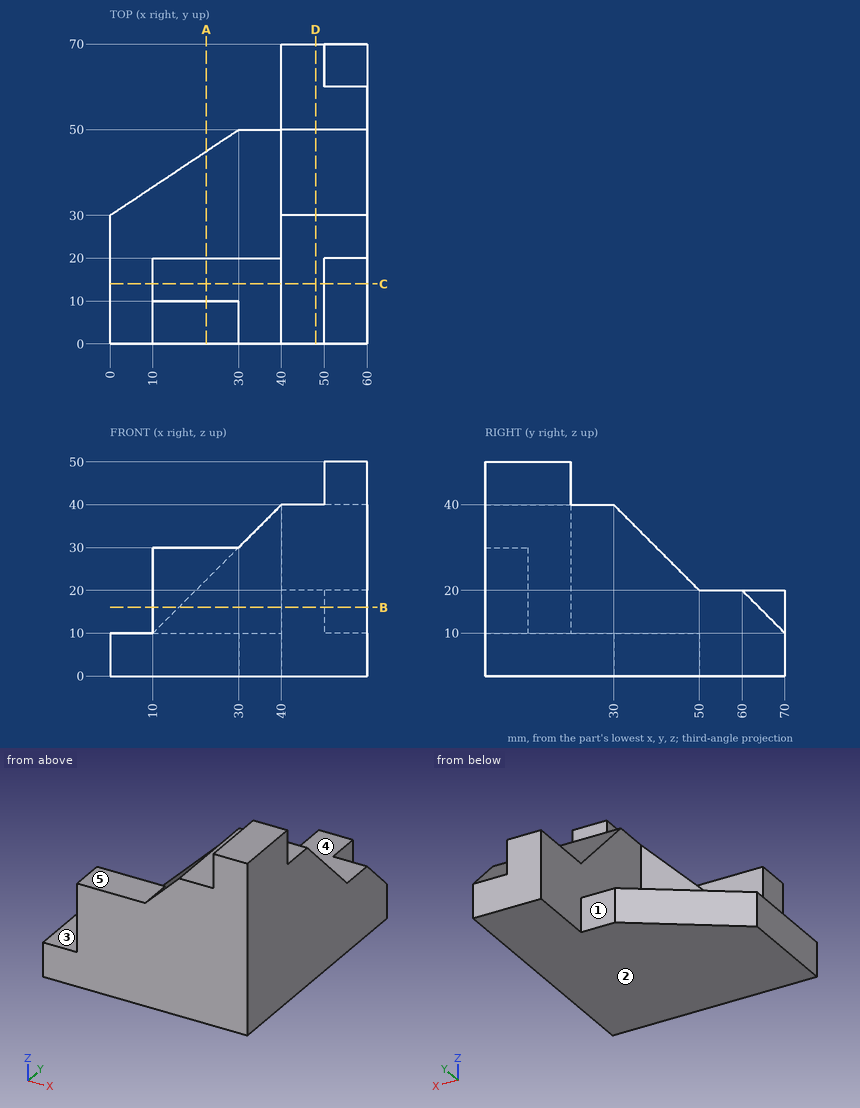
Can you work these out from the drawing? Everything is in mm from the part's minimum corner. A direction names the side the tool comes from. Round coordinates to 2 decimals unless told otherwise and drop trailing zeros. Order: outer loops, then holes, each group sorted by start corner. A loop starts at its lowest first (then second) coordinate and runs counter-clockwise, first axis right, second up. Notation, with made-up numbers: M 1.25,55.5 L 46.25,55.5 A26 ccw 46.25,78.5 Z; hole C -17,65.25 d10. An arc over 180 degrees is marked long. One line per question, with ' | ' between items.
1) For the marked faces 1, 2, 3, 4 and 5, which set-ups out of +Z, -Z, +X, -X, +Y, -Y let a thin tool reach every point of the face, with its end or its side?
Working result:
face 1: +Z, -Z, -X, +Y | face 2: -Z, +X, -X, +Y, -Y | face 3: +Z, -X, +Y | face 4: +Z, +X, -X, +Y | face 5: +Z, -X, +Y, -Y
2) I want a section at D-D, the plane x = 48. Write out the boundary of the cut face in (y, z), then the cut area to 3 significant figures.
Working result:
outline: M 0,0 L 70,0 L 70,20 L 50,20 L 30,40 L 0,40 Z | area: 2,200 mm²
3) I want a section at C-C, the plane y = 14. Write out the boundary of the cut face in (x, z), then the cut area to 3 significant figures.
Working result:
outline: M 0,0 L 60,0 L 60,50 L 50,50 L 50,40 L 40,40 L 10,10 L 0,10 Z | area: 1,750 mm²
4) I want a section at B-B, the plane z = 16. Write out the boundary of the cut face in (x, y), then the cut area to 3 significant figures.
Working result:
outline: M 10,0 L 60,0 L 60,64 L 50,64 L 50,70 L 40,70 L 40,20 L 16,20 L 16,10 L 10,10 Z | area: 1,880 mm²
5) For pin 1 Ø5 at (x, z) = (57.5, 43.5) entering from +Y; pin 2 Ø2 at (x, z) = (14, 8) entering from +Y; pin 3 Ø1 at (y, z) = (42.5, 16) entering from -X, each with a flat end and sliding along its axis, tell me the tip position at first contact or that it passes through.
Working result:
pin 1: y = 20 | pin 2: y = 40 | pin 3: x = 40
6) I want a section at A-A, the plane x = 22.5. Write out the boundary of the cut face in (y, z), then the cut area to 3 significant figures.
Working result:
outline: M 0,0 L 45,0 L 45,10 L 20,10 L 20,22.5 L 10,22.5 L 10,30 L 0,30 Z | area: 775 mm²
7) I need wall thicknesses on line 1 along X through (y, z) = (42, 21); line 2 along Z through (x, y) = (44, 28); line 3 along Z through (x, y) = (57.5, 60). Which ranges of each line are inside material? Lowest first, please.
Working result:
line 1: 40 to 60 | line 2: 0 to 40 | line 3: 0 to 20
